Design review of the part built by this model. Coordinates are the model's own, in mm. A direction names the side the tool comes from. Coordinates: 2 decimals unless noted, no trailing zeros. Write each loop counter-clockwise with the first axis right and the second up, starting at its lowest first coordinate (ties: lowest second). Pieces come first, ordered by that corner, then holes. Notation, with made-up numbers: (73.25, -27) - (123.25, -27) arc R32 ccw to (123.25, 10) - close; hole circle Ø3 at (75.25, -17). An arc over 180 degrees is marked (long way). Answer as a JSON object with one key per item and string values.
```python
from build123d import *

# Parameters (mm, degrees)
F1_DEPTH = 147.32


with BuildPart() as f1:
    # F0 (on Front) → F1 (new body)
    with BuildSketch(Plane.XZ):
        Polygon((-212.958432, 62.320832), (-306.938432, 62.320832), (-306.938432, 1.360832), (74.061568, 1.360832), (74.061568, 62.320832), (-19.918432, 62.320832), align=None)
        with BuildLine():
            Line((-212.958432, 128.360832), (-212.958432, 62.320832))
            Line((-212.958432, 62.320832), (-19.918432, 62.320832))
            Line((-19.918432, 62.320832), (-19.918432, 128.360832))
            Line((-19.918432, 128.360832), (-51.668432, 128.360832))
            ThreePointArc((-51.668432, 128.360832), (-116.438432, 75.209924), (-181.208432, 128.360832))
            Line((-181.208432, 128.360832), (-212.958432, 128.360832))
        make_face()
    extrude(amount=F1_DEPTH)


solid = f1.part
```
(1) To check wall thickness, follow line 1 (Z direction, x = 2, y = -37); line 2 (X direction, y = -70, z = 84); line 3 (X direction, y = -82.5, z = 82). State the ranges of each line that lie inside material, in increasing order. Write a range as from..to.
Solved:
{"line 1": "z = 1.36..62.32", "line 2": "x = -212.96..-149.36, -83.52..-19.92", "line 3": "x = -212.96..-145.61, -87.27..-19.92"}
(2) For pin 1 (12 mm diameter, centred on y = -16.5, z = 104.5, fed in from -X); pin 2 (6 mm diameter, centred on y = -105, z = 74.5, fed in from +X), all flat-tipped, find the tip position at first contact; note any pin that passes through.
Solved:
{"pin 1": "stops at x = -212.96", "pin 2": "stops at x = -19.92"}
(3) Take a section at D-D, the plane x = -90. Write out the cut boundary in (y, z).
Solved:
{"outline": "(-147.32, 1.36) - (0, 1.36) - (0, 80.73) - (-147.32, 80.73) - close"}
(4) Take a section at C-C, the plane x = 32.5. Write out the cut boundary in (y, z), and give its area (3 significant figures).
Solved:
{"outline": "(-147.32, 1.36) - (0, 1.36) - (0, 62.32) - (-147.32, 62.32) - close", "area": "8,980 mm^2"}
(5) Take a section at B-B, the plane z = 98. Write out the cut boundary in (x, y), and give its area (3 significant figures).
Solved:
{"outline": "(-212.96, -147.32) - (-166.35, -147.32) - (-166.35, 0) - (-212.96, 0) - close; (-66.53, -147.32) - (-19.92, -147.32) - (-19.92, 0) - (-66.53, 0) - close", "area": "13,700 mm^2"}
(6) Take a section at A-A, the plane y = -63.5. Write out the cut boundary in (x, z).
Solved:
{"outline": "(-306.94, 1.36) - (74.06, 1.36) - (74.06, 62.32) - (-19.92, 62.32) - (-19.92, 128.36) - (-51.67, 128.36) arc R66.04 cw to (-181.21, 128.36) - (-212.96, 128.36) - (-212.96, 62.32) - (-306.94, 62.32) - close"}
(7) The part is to be moulded in two halves that separate along X. For faces 4 (the face through (-119, -147.32, 52)), 5 (the face through (74.062, -73, 31)), 6 (the face through (-115.168, -72.629, 75.222)), say which applies: pulls with the +X half, pulls with the -X half, needs draft (parallel to the pull), parting line crosses it, or undercut.
Solved:
{"face 4": "needs draft", "face 5": "pulls with the +X half", "face 6": "undercut"}
(8) Tool access review of faces 1 (the face through (-212.958, -73, 96)), 2 (the face through (28, -73, 62.321)), 3 (the face through (-197, -73, 128.361)): name each direction out of +Z, -Z, +X, -X, +Y, -Y from which nothing blocks a thin tool from reaching the whole face with its end or side.
Solved:
{"face 1": "+Z, -X, +Y, -Y", "face 2": "+Z, +X, +Y, -Y", "face 3": "+Z, +X, -X, +Y, -Y"}
